Input: dimensioned drawing with shaded views. Units: mm. Origin: part minimum x, y, z. Give positions to 0.01 mm unless a question says otherwise; leave off trailing zeros. Write each loop counter-clockwise with the first axis right and the second up, starting at its lowest first coordinate (ties: lowest second). Pieces come first, ordered by that corner, then holes.
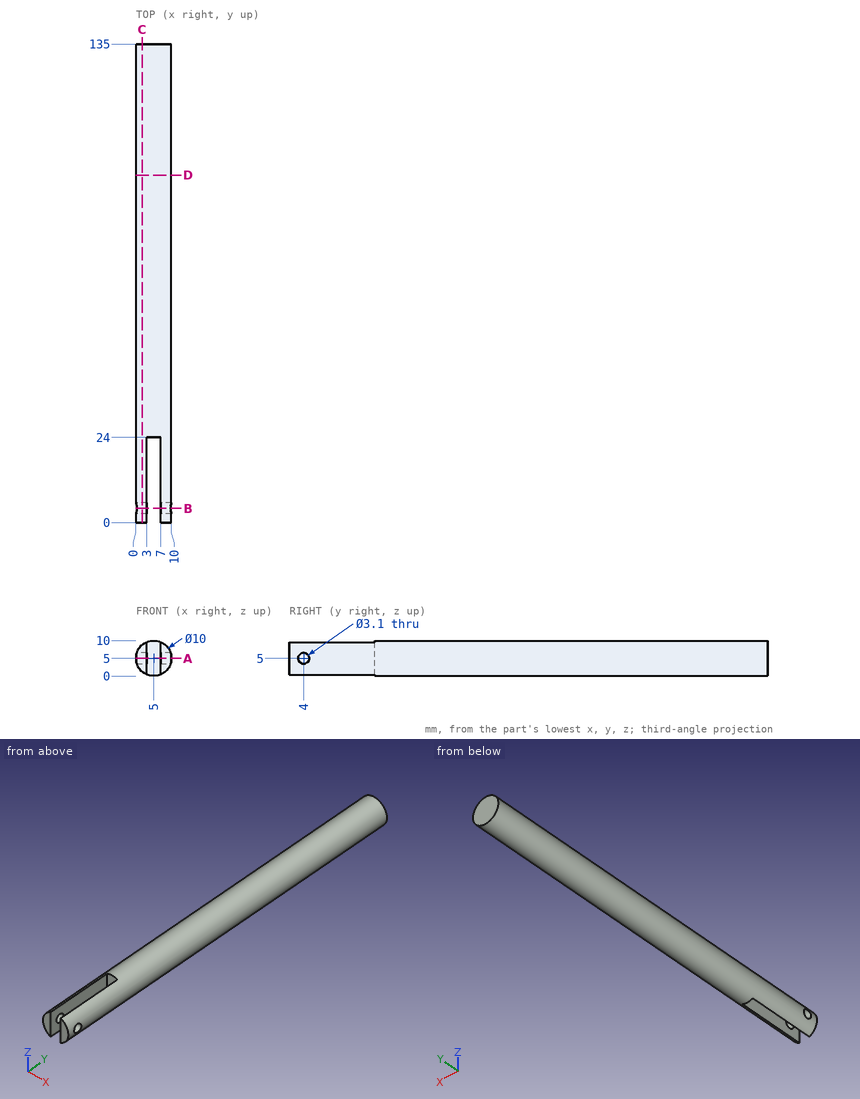
1. Line query: L1, parallel to Y at x = 7.6, z = 5; L2, parallel to Y at x = 7.75, z = 4; L3, parallel to X at y = 71, z = 5.5. Output: solid intervals per line, ascending.
2. Cut plane A-A, the plane z = 5. Return the cut outline in (x, y).
3. Cut plane D-D, the plane y = 98. Return the cut outline in (x, z).
4. Contact query for flat-ended pins moving along their axis: P1, Ø2, axis at x = 4.5, z = 6.5, coming from the -Y side; P2, Ø1, axis at x = 6, y = 27.5, coming from the +Z side; P3, Ø4, axis at y = 117.5, z = 7.5, coming from the +X side. Output: stop coordinate, or through.
5. Cut plane C-C, the plane x = 1.75. Return the cut outline in (y, z).
6. Cut plane B-B, the plane y = 4. Return the cut outline in (x, z).
Response values:
1. L1: y = 0 to 2.45, 5.55 to 135
1. L2: y = 0 to 2.82, 5.18 to 135
1. L3: x = 0.03 to 9.97
2. outline: (0, 0) - (3, 0) - (3, 2.45) - (0, 2.45) - close; (0, 5.55) - (3, 5.55) - (3, 24) - (7, 24) - (7, 5.55) - (10, 5.55) - (10, 135) - (0, 135) - close; (7, 0) - (10, 0) - (10, 2.45) - (7, 2.45) - close
3. outline: circle Ø10 at (5, 5)
4. P1: stops at y = 24
4. P2: stops at z = 9.97
4. P3: stops at x = 9.97
5. outline: (0, 1.2) - (135, 1.2) - (135, 8.8) - (0, 8.8) - close; hole circle Ø3.1 at (4, 5)
6. outline: (0.25, 3.45) arc R5 ccw to (3, 0.42) - (3, 3.45) - close; (0.25, 6.55) - (3, 6.55) - (3, 9.58) arc R5 ccw to start; (7, 0.42) arc R5 ccw to (9.75, 3.45) - (7, 3.45) - close; (7, 6.55) - (9.75, 6.55) arc R5 ccw to (7, 9.58) - close
